```python
from build123d import *

# Parameters (mm, degrees)
SKETCH1_W            = 62
SKETCH1_H            = 61.770504471
SKETCH1_R            = 4
SKETCH1_R_2          = 27.5
SKETCH1_R_3          = 2
SKETCH1_R_4          = 22.5
BOSS_EXTRUDE6_DEPTH  = 8
SKETCH1_15_W         = 78
SKETCH1_15_H         = 77.770504471
SKETCH1_15_W_2       = 62
SKETCH1_15_H_2       = 61.770504471
BOSS_EXTRUDE9_DEPTH  = 69
SKETCH1_17_R         = 4
CUT_EXTRUDE2_DEPTH   = 56
SKETCH1_18_R         = 4
SKETCH1_18_R_2       = 2
BOSS_EXTRUDE10_DEPTH = 4
CUT_EXTRUDE10_DEPTH  = 8
CUT_EXTRUDE11_DEPTH  = 8
SKETCH6_W            = 21
SKETCH6_H            = 37
CUT_EXTRUDE13_DEPTH  = 10
SKETCH12_W           = 77.770504471
SKETCH12_H           = 20
BOSS_EXTRUDE12_DEPTH = 80
BOSS_EXTRUDE13_DEPTH = 10
SKETCH14_W           = 3
SKETCH14_H           = 78.415811308
BOSS_EXTRUDE14_DEPTH = 3
SKETCH15_R           = 25.5
CUT_EXTRUDE14_DEPTH  = 15
FILLET1_R            = 10


with BuildPart() as part:
    # Sketch1 → Boss-Extrude6 (new body)
    # profile 1 of 11: a face of its own
    with BuildSketch(Plane(origin=(0, 0, 0), x_dir=(1, 0, 0), z_dir=(0, 1, 0))):
        with Locations((31, 30.885252236)):
            Rectangle(SKETCH1_W, SKETCH1_H)
        with Locations((56.343145751, 56.113650222)):
            Circle(SKETCH1_R, mode=Mode.SUBTRACT)
        with Locations((31, 31)):
            Circle(SKETCH1_R_2, mode=Mode.SUBTRACT)
        with Locations((5.656854249, 56.113650222)):
            Circle(SKETCH1_R, mode=Mode.SUBTRACT)
        with Locations((56.343145751, 5.656854249)):
            Circle(SKETCH1_R, mode=Mode.SUBTRACT)
        with Locations((5.656854249, 5.656854249)):
            Circle(SKETCH1_R, mode=Mode.SUBTRACT)
    # profile 2 of 11: a face of its own
    with BuildSketch(Plane(origin=(0, 0, 0), x_dir=(1, 0, 0), z_dir=(0, 1, 0))):
        with Locations((5.656854249, 5.656854249)):
            Circle(SKETCH1_R)
        with Locations((5.656854249, 5.656854249)):
            Circle(SKETCH1_R_3, mode=Mode.SUBTRACT)
    # profile 3 of 11: a face of its own
    with BuildSketch(Plane(origin=(0, 0, 0), x_dir=(1, 0, 0), z_dir=(0, 1, 0))):
        with Locations((5.656854249, 5.656854249)):
            Circle(SKETCH1_R_3)
    # profile 4 of 11: a face of its own
    with BuildSketch(Plane(origin=(0, 0, 0), x_dir=(1, 0, 0), z_dir=(0, 1, 0))):
        with Locations((56.343145751, 5.656854249)):
            Circle(SKETCH1_R)
        with Locations((56.343145751, 5.656854249)):
            Circle(SKETCH1_R_3, mode=Mode.SUBTRACT)
    # profile 5 of 11: a face of its own
    with BuildSketch(Plane(origin=(0, 0, 0), x_dir=(1, 0, 0), z_dir=(0, 1, 0))):
        with Locations((56.343145751, 5.656854249)):
            Circle(SKETCH1_R_3)
    # profile 6 of 11: a face of its own
    with BuildSketch(Plane(origin=(0, 0, 0), x_dir=(1, 0, 0), z_dir=(0, 1, 0))):
        with Locations((56.343145751, 56.113650222)):
            Circle(SKETCH1_R)
        with Locations((56.343145751, 56.113650222)):
            Circle(SKETCH1_R_3, mode=Mode.SUBTRACT)
    # profile 7 of 11: a face of its own
    with BuildSketch(Plane(origin=(0, 0, 0), x_dir=(1, 0, 0), z_dir=(0, 1, 0))):
        with Locations((56.343145751, 56.113650222)):
            Circle(SKETCH1_R_3)
    # profile 8 of 11: a face of its own
    with BuildSketch(Plane(origin=(0, 0, 0), x_dir=(1, 0, 0), z_dir=(0, 1, 0))):
        with Locations((5.656854249, 56.113650222)):
            Circle(SKETCH1_R)
        with Locations((5.656854249, 56.113650222)):
            Circle(SKETCH1_R_3, mode=Mode.SUBTRACT)
    # profile 9 of 11: a face of its own
    with BuildSketch(Plane(origin=(0, 0, 0), x_dir=(1, 0, 0), z_dir=(0, 1, 0))):
        with Locations((5.656854249, 56.113650222)):
            Circle(SKETCH1_R_3)
    # profile 10 of 11: a face of its own
    with BuildSketch(Plane(origin=(0, 0, 0), x_dir=(1, 0, 0), z_dir=(0, 1, 0))):
        with Locations((31, 31)):
            Circle(SKETCH1_R_2)
        with Locations((31, 31)):
            Circle(SKETCH1_R_4, mode=Mode.SUBTRACT)
    # profile 11 of 11: a face of its own
    with BuildSketch(Plane(origin=(0, 0, 0), x_dir=(1, 0, 0), z_dir=(0, 1, 0))):
        with Locations((31, 31)):
            Circle(SKETCH1_R_4)
    extrude(amount=BOSS_EXTRUDE6_DEPTH)

    # Sketch1_15 → Boss-Extrude9 (add)
    with BuildSketch(Plane(origin=(0, 0, 0), x_dir=(1, 0, 0), z_dir=(0, 1, 0))):
        with Locations((31, 30.885252236)):
            Rectangle(SKETCH1_15_W, SKETCH1_15_H)
        with Locations((31, 30.885252236)):
            Rectangle(SKETCH1_15_W_2, SKETCH1_15_H_2, mode=Mode.SUBTRACT)
    extrude(amount=BOSS_EXTRUDE9_DEPTH)

    # Sketch1_17 → Cut-Extrude2 (cut)
    with BuildSketch(Plane(origin=(0, 0, 0), x_dir=(1, 0, 0), z_dir=(0, 1, 0))):
        with Locations(Location((5.656854249, 56.113650222, 0), (0, 0, 270))):
            Circle(SKETCH1_17_R)
        with Locations(Location((56.343145751, 56.113650222, 0), (0, 0, 90))):
            Circle(SKETCH1_17_R)
        with Locations(Location((56.343145751, 5.656854249, 0), (0, 0, 270))):
            Circle(SKETCH1_17_R)
        with Locations(Location((5.656854249, 5.656854249, 0), (0, 0, 90))):
            Circle(SKETCH1_17_R)
    extrude(amount=CUT_EXTRUDE2_DEPTH, mode=Mode.SUBTRACT)

    # Sketch1_18 → Boss-Extrude10 (add)
    # profile 1 of 4: a face of its own
    with BuildSketch(Plane(origin=(0, 0, 0), x_dir=(1, 0, 0), z_dir=(0, 1, 0))):
        with Locations(Location((5.656854249, 56.113650222, 0), (0, 0, 270))):
            Circle(SKETCH1_18_R)
        with Locations(Location((5.656854249, 56.113650222, 0), (0, 0, 270))):
            Circle(SKETCH1_18_R_2, mode=Mode.SUBTRACT)
    # profile 2 of 4: a face of its own
    with BuildSketch(Plane(origin=(0, 0, 0), x_dir=(1, 0, 0), z_dir=(0, 1, 0))):
        with Locations(Location((56.343145751, 56.113650222, 0), (0, 0, 90))):
            Circle(SKETCH1_18_R)
        with Locations(Location((56.343145751, 56.113650222, 0), (0, 0, 90))):
            Circle(SKETCH1_18_R_2, mode=Mode.SUBTRACT)
    # profile 3 of 4: a face of its own
    with BuildSketch(Plane(origin=(0, 0, 0), x_dir=(1, 0, 0), z_dir=(0, 1, 0))):
        with Locations(Location((56.343145751, 5.656854249, 0), (0, 0, 270))):
            Circle(SKETCH1_18_R)
        with Locations(Location((56.343145751, 5.656854249, 0), (0, 0, 270))):
            Circle(SKETCH1_18_R_2, mode=Mode.SUBTRACT)
    # profile 4 of 4: a face of its own
    with BuildSketch(Plane(origin=(0, 0, 0), x_dir=(1, 0, 0), z_dir=(0, 1, 0))):
        with Locations(Location((5.656854249, 5.656854249, 0), (0, 0, 90))):
            Circle(SKETCH1_18_R)
        with Locations(Location((5.656854249, 5.656854249, 0), (0, 0, 90))):
            Circle(SKETCH1_18_R_2, mode=Mode.SUBTRACT)
    extrude(amount=BOSS_EXTRUDE10_DEPTH)

    # Sketch3 → Cut-Extrude10 (cut)
    with BuildSketch(Plane(origin=(0, 0, -69.770504471), x_dir=(-1, 0, 0), z_dir=(0, 0, -1))):
        Polygon((-42.5, 69), (-42.5, 64), (-19.5, 65), (-19.5, 69), align=None)
    extrude(amount=-CUT_EXTRUDE10_DEPTH, mode=Mode.SUBTRACT)

    # Sketch9 → Cut-Extrude11 (cut)
    with BuildSketch(Plane.XY.offset(8)):
        Polygon((19.5, 69), (19.5, 64), (42.5, 65), (42.5, 69), align=None)
    extrude(amount=-CUT_EXTRUDE11_DEPTH, mode=Mode.SUBTRACT)

    # Sketch6 → Cut-Extrude13 (cut)
    with BuildSketch(Plane.ZY.offset(8)):
        with Locations((-30.885252236, 50.5)):
            Rectangle(SKETCH6_W, SKETCH6_H)
    extrude(amount=-CUT_EXTRUDE13_DEPTH, mode=Mode.SUBTRACT)

    # Sketch12 → Boss-Extrude12 (add)
    with BuildSketch(Plane(origin=(70, 0, 0), x_dir=(0, 0, -1), z_dir=(1, 0, 0))):
        with Locations((30.885252236, 10)):
            Rectangle(SKETCH12_W, SKETCH12_H)
    extrude(amount=BOSS_EXTRUDE12_DEPTH)

    # Sketch13 → Boss-Extrude13 (add)
    with BuildSketch(Plane(origin=(70, 0, 0), x_dir=(0, 0, -1), z_dir=(1, 0, 0))):
        Polygon((-8, 59.539327542), (69.770504471, 49.5), (69.770504471, 44.5), (-8, 54.539327542), align=None)
    extrude(amount=BOSS_EXTRUDE13_DEPTH)

    # Sketch14 → Boss-Extrude14 (add)
    with BuildSketch(Plane(origin=(0, 57.547640196, -7.428775384), x_dir=(1, 0, 0), z_dir=(0, 0.9917707050815963, -0.12802682743063418))):
        with Locations((78.5, 23.651108801)):
            Rectangle(SKETCH14_W, SKETCH14_H)
    extrude(amount=BOSS_EXTRUDE14_DEPTH)

    # Sketch15 → Cut-Extrude14 (cut)
    with BuildSketch(Plane(origin=(0, 20, 0), x_dir=(1, 0, 0), z_dir=(0, 1, 0))):
        with Locations(Location((114.5, 30.885252236, 0), (0, 0, 270))):
            Circle(SKETCH15_R)
    extrude(amount=-CUT_EXTRUDE14_DEPTH, mode=Mode.SUBTRACT)

    # Fillet1
    fillet1_edges = [part.edges().sort_by_distance(p)[0] for p in [
        (150, 10, 8),
        (150, 10, -69.770504471),
        (-8, 34.5, 8),
        (-8, 34.5, -69.770504471),
    ]]
    fillet(fillet1_edges, radius=FILLET1_R)


solid = part.part
```
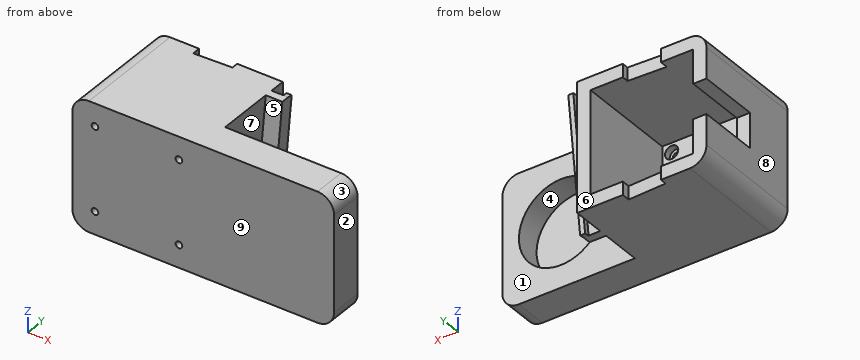
For this review, take the finished solid that the model builds, in its own axes (mm). Face numbers are marked on the shaded views. A direction names the side the tool comes from. Round coordinates to 2 decimals unless told otherwise and drop trailing zeros. Write each loop counter-clockwise with the first axis right and the second up, starting at its lowest first coordinate (ties: lowest second). Pieces come first, ordered by that corner, then holes. Notation, with made-up numbers: (9, 58) - (63, 58) arc R24 cw to (63, 81) - close; hole circle Ø3 at (-35.5, -13). An arc over 180 degrees is marked (long way). Write each question's results on one line, items separated by ' | '.
Item 1: Take a section at B-B on y = 39.5. State the section outline as (x, z) points.
Calculated:
outline: (-8, -59.77) arc R10 ccw to (2, -69.77) - (70, -69.77) - (70, 8) - (2, 8) arc R10 ccw to (-8, -2) - (-8, -20.39) - (0, -20.39) - (0, 0) - (62, 0) - (62, -61.77) - (0, -61.77) - (0, -41.39) - (-8, -41.39) - close
Item 2: Draft analysis for pull direction Y (two halves, no side actions). For the marked faces 6, 7, 8 and 9, state which applies: pulls with the +Y half, pulls with the -Y half, needs draft (parallel to the pull), parting line crosses it, or undercut.
Calculated:
face 6: pulls with the +Y half | face 7: undercut | face 8: needs draft | face 9: pulls with the -Y half
Item 3: Take a section at C-C on z = -18. State the section outline as (x, y) points (3 decimals).
Calculated:
outline: (-8, 0) - (150, 0) - (150, 20) - (136.505, 20) - (136.505, 5) - (92.495, 5) - (92.495, 20) - (70, 20) - (70, 51.183) - (80, 51.183) - (80, 59.208) - (77, 59.208) - (77, 56.183) - (70, 56.183) - (70, 69) - (62, 69) - (62, 8) - (0, 8) - (0, 69) - (-8, 69) - close
Item 4: Take a section at D-D on x = 15. State the section outline as (y, z) points, then the cut area to 3 significant figures.
Calculated:
outline: (0, -69.77) - (69, -69.77) - (69, -61.77) - (8, -61.77) - (8, 0) - (69, 0) - (69, 8) - (0, 8) - close | area: 1,600 mm^2
Item 5: For pin 1 (2 mm diameter, centred on y = 67, z = -67, fed in from +X); pin 2 (1 mm diameter, centred on x = 111, z = -45, fed in from +Y); pin 3 (4 mm diameter, centred on x = 50, z = -29.5, fed in from +Y); pin 4 (2.5 mm diameter, centred on x = 56.34, z = -56.11, fed in from +Y), all flat-tipped, find the tip position at first contact; note any pin that passes through.
Calculated:
pin 1: stops at x = 70 | pin 2: stops at y = 5 | pin 3: stops at y = 8 | pin 4: passes through
Item 6: Take a section at A-A on x = 114.5. State the section outline as (y, z) points.
Calculated:
outline: (0, -69.77) - (20, -69.77) - (20, -56.39) - (5, -56.39) - (5, -5.39) - (20, -5.39) - (20, 8) - (0, 8) - close
Item 7: To check wall thickness, follow line 1 along X through (y, z) = (53, -52.5); line 2 along Z through (x, y) = (28.5, 14); line 3 along Z through (x, y) = (114, 11). State the ranges of each line that lie inside material, in increasing order. Write a range as from..to.
Calculated:
line 1: x = -8..0, 62..70, 77..80 | line 2: z = -69.77..-61.77, 0..8 | line 3: z = -69.77..-56.38, -5.39..8
Item 8: For the marked faces 1, 2, 3, 4 and 5, list the 3-axis set-ups (+Z, -Z, +X, -X, +Y, -Y) from which the entire face can be reached by the end or side of a thin tool; tool diameter is ignored.
Calculated:
face 1: +Z, -Z, +X | face 2: +Z, -Z, +X, +Y, -Y | face 3: +Z, +X, +Y, -Y | face 4: +Y | face 5: +Z, +X
